Part model, mm, in its own coordinate system. A direction names the side the tool comes from. Give positions to 0.01 mm unless a question says otherwise; leave off trailing zeros. Order: outer loops, then holes, each group sorted by start corner. A loop starts at its lowest first (then second) coordinate and runs counter-clockwise, first axis right, second up. Notation, with made-up numbers: M -16.75,12 L 27.25,12 A27 ccw 27.25,42 Z; hole C -3.5,52 d3. An arc over 180 degrees is marked long. One line per question, with ' | ' between items.
```python
from build123d import *

# Parameters (mm, degrees)
SKETCH1_R           = 10
SKETCH1_R_2         = 1.5
SKETCH1_R_3         = 4.75
SKETCH1_R_4         = 2.9
BOSS_EXTRUDE1_DEPTH = 2
SKETCH1_3_R         = 4.75
SKETCH1_3_R_2       = 2.9
BOSS_EXTRUDE2_DEPTH = 3


with BuildPart() as part:
    # Sketch1 → Boss-Extrude1 (new body)
    # profile 1 of 3: a face of its own
    with BuildSketch(Plane(origin=(0, 0, 0), x_dir=(1, 0, 0), z_dir=(0, 1, 0))):
        with Locations(Location((0, 0, 0), (0, 0, 270))):
            Circle(SKETCH1_R)
        with Locations(Location((7, 0, 0), (0, 0, 270))):
            Circle(SKETCH1_R_2, mode=Mode.SUBTRACT)
        with Locations(Location((0, 7, 0), (0, 0, 270))):
            Circle(SKETCH1_R_2, mode=Mode.SUBTRACT)
        with Locations(Location((-7, 0, 0), (0, 0, 270))):
            Circle(SKETCH1_R_2, mode=Mode.SUBTRACT)
        with Locations(Location((0, -7, 0), (0, 0, 270))):
            Circle(SKETCH1_R_2, mode=Mode.SUBTRACT)
        Circle(SKETCH1_R_3, mode=Mode.SUBTRACT)
    # profile 2 of 3: a face of its own
    with BuildSketch(Plane(origin=(0, 0, 0), x_dir=(1, 0, 0), z_dir=(0, 1, 0))):
        Circle(SKETCH1_R_3)
        Circle(SKETCH1_R_4, mode=Mode.SUBTRACT)
    # profile 3 of 3: a face of its own
    with BuildSketch(Plane(origin=(0, 0, 0), x_dir=(1, 0, 0), z_dir=(0, 1, 0))):
        Circle(SKETCH1_R_4)
        with Locations(Location((0, 0, 0), (0, 0, 270))):
            Circle(SKETCH1_R_2, mode=Mode.SUBTRACT)
    extrude(amount=BOSS_EXTRUDE1_DEPTH)

    # Sketch1_3 → Boss-Extrude2 (add)
    with BuildSketch(Plane(origin=(0, 0, 0), x_dir=(1, 0, 0), z_dir=(0, 1, 0))):
        with Locations(Location((0, 0, 0), (0, 0, 270))):
            Circle(SKETCH1_3_R)
        with Locations(Location((0, 0, 0), (0, 0, 270))):
            Circle(SKETCH1_3_R_2, mode=Mode.SUBTRACT)
    extrude(amount=-BOSS_EXTRUDE2_DEPTH)


solid = part.part
```
1. Probe L1, parallel to X at y = 1, z = 0; L2, parallel to X at y = -2.2, z = 0; L3, parallel to X at y = 1.6, z = -0.5. List the from-to ranges inside material, lowest first. Write a range as from..to.
Worked out:
L1: x = -10..-8.5, -5.5..-1.5, 1.5..5.5, 8.5..10 | L2: x = -4.75..-2.9, 2.9..4.75 | L3: x = -9.99..-8.41, -5.59..-1.41, 1.41..5.59, 8.41..9.99
2. Slice it at B-B on x = 0. Give the cut face in (y, z).
Worked out:
outline: M -3,-4.75 L 0,-4.75 L 0,-5.5 L 2,-5.5 L 2,-1.5 L 0,-1.5 L 0,-2.9 L -3,-2.9 Z; M -3,2.9 L 0,2.9 L 0,1.5 L 2,1.5 L 2,5.5 L 0,5.5 L 0,4.75 L -3,4.75 Z; M 0,-10 L 2,-10 L 2,-8.5 L 0,-8.5 Z; M 0,8.5 L 2,8.5 L 2,10 L 0,10 Z
3. Tool access for faces 4 (the cylindrical face through (0.45, 0.99, 1.43)), 5 (the flat face through (1.2, 0, 1.2)): list every direction of +Z, -Z, +X, -X, +Y, -Y with a clear straight run to the whole face (end or side of a thin tool).
Worked out:
face 4: +Y, -Y | face 5: -Y
4. Slice it at C-C on x = -7. Give the cut face in (y, z), then the cut area to 3 significant figures.
Worked out:
outline: M 0,-7.14 L 2,-7.14 L 2,-1.5 L 0,-1.5 Z; M 0,1.5 L 2,1.5 L 2,7.14 L 0,7.14 Z | area: 22.6 mm2
5. Slice it at D-D on y = 1. Give the cut face in (x, z), then the cut area to 3 significant figures.
Worked out:
outline: C 0,0 d20; hole C -7,0 d3; hole C 0,-7 d3; hole C 0,0 d3; hole C 0,7 d3; hole C 7,0 d3 | area: 279 mm2
6. Drop flat-ended pins along their axis: pin 1 (2 mm diameter, centred on x = 2, y = -0.5, fed in from -Z); pin 2 (3 mm diameter, centred on y = -2, z = 6.5, fed in from +X); pin 3 (3.5 mm diameter, centred on x = 0, z = 7, fed in from -Y); pin 4 (1.5 mm diameter, centred on x = 7, y = 1, fed in from +Z). Give the stop position or say it passes through.
Worked out:
pin 1: stops at z = -9.94 | pin 2: passes through | pin 3: stops at y = 0 | pin 4: stops at z = 7.81
7. Mould opens along Z. For faces 1 (the flat face through (4.3, 0, -2.4)), 2 (the cylindrical face through (0.1, -1.5, -2.9)), 3 (the cylindrical face through (-2.89, -1.48, -3.77)) say: released by +Z, released by -Z, zero draft, split by the parting line, or undercut.
Worked out:
face 1: zero draft | face 2: undercut | face 3: split by the parting line
8. Slice it at A-A on z = 0. Give the cut face in (x, y).
Worked out:
outline: M -10,0 L -8.5,0 L -8.5,2 L -10,2 Z; M -5.5,0 L -4.75,0 L -4.75,-3 L -2.9,-3 L -2.9,0 L -1.5,0 L -1.5,2 L -5.5,2 Z; M 1.5,0 L 2.9,0 L 2.9,-3 L 4.75,-3 L 4.75,0 L 5.5,0 L 5.5,2 L 1.5,2 Z; M 8.5,0 L 10,0 L 10,2 L 8.5,2 Z
